Autodesk Inventor part; units mm, degrees
ref_plane "YZ Plane" through (0, 0, 0) normal (1, 0, 0) x (0, 1, 0)
ref_plane "XZ Plane" through (0, 0, 0) normal (0, 1, 0) x (-1, 0, 0)
ref_plane "XY Plane" through (0, 0, 0) normal (0, 0, 1) x (1, 0, 0)
sketch "Sketch1" plane through (0, 0, 0) normal (0, 1, 0) x (-1, 0, 0)
  line L0 (214.6102, -0.0199) -> (304.9164, -0.0199)
  line L1 (304.9164, -0.0199) -> (214.6102, -0.0199)
  line L2 (304.9164, -0.0199) -> (127, -1041.4)
  line L3 (127, -1041.4) -> (38.2671, -1041.4)
  line L4 (39.368, -1026.4384) -> (214.6102, -0.0199)
  line L5 (38.2671, -1041.4) -> (36.8136, -1041.4)
  line L6 (39.368, -1026.4384) -> (36.8136, -1041.4)
  point P0 (0, 0)
extrude "Extrusion1" add sketch "Sketch1" along normal blind 38.1
properties part number "S_2x4x48.76"
CAD build for the part. Positions are in the model's coordinates, mm. Give positions to 0.01 mm unless a question says otherwise; leave off trailing zeros. Loops run counter-clockwise (first coordinate to the right, second up) from the corner with the lowest first, then second, coordinate; pieces in that order, holes last. Notation, with made-up numbers: M 63,-11.75 L 87,-11.75 A32 ccw 87,20.25 Z; hole C 2,-27.5 d7. An arc over 180 degrees is marked long. Answer in a Markdown table with one row per item. Add a question column.
Item 1: Probe probe 1 along X at (y, z) = (35, -414); probe 2 along X at (y, z) = (15.5, -863). List the from-to ranges inside material, lowest first.
Item 2: Mould opens along Z. For faces 1 (the face through (-217.204, 18.783, -513.42)), 2 (the face through (-150, 0, -518)), 3 (the face through (-259, 19, -0.02)) say: +Z half, -Z half, draft (parallel to the pull), parting line (faces both ways), or undercut.
Item 3: Band-saw the part on C-C on x = -94. Give the cut face in (y, z), then the cut area to 3 significant figures.
Item 4: Band-saw the part on A-A on y = 23. Give the cut face in (x, z), then the cut area to 3 significant figures.
Item 5: Band-saw the part on B-B on z = -615. Give the cut face in (x, y).
Item 6: Drop flat-ended pins along their axis: P1, Ø1.5, axis at y = 23.5, z = -214, coming from the -X side; P2, Ø4, axis at y = 6, z = -165.5, coming from the +X side; P3, Ø3, axis at y = 22.5, z = -325, coming from the -X side. Give the stop position or say it passes through.
Reply:
| question | item | result |
|---|---|---|
| 1 | probe 1 | x = -234.19 to -143.93 |
| 1 | probe 2 | x = -157.48 to -67.27 |
| 2 | face 1 | -Z half |
| 2 | face 2 | draft |
| 2 | face 3 | +Z half |
| 3 | outline | M 0,-1041.4 L 38.1,-1041.4 L 38.1,-706.45 L 0,-706.45 Z |
| 3 | area | 12,800 mm^2 |
| 4 | outline | M -304.92,-0.02 L -127,-1041.4 L -36.81,-1041.4 L -39.37,-1026.44 L -214.61,-0.02 Z |
| 4 | area | 94,000 mm^2 |
| 5 | outline | M -199.85,0 L -109.61,0 L -109.61,38.1 L -199.85,38.1 Z |
| 6 | P1 | stops at x = -268.49 |
| 6 | P2 | stops at x = -186.02 |
| 6 | P3 | stops at x = -249.65 |
